```python
from build123d import *

# Parameters (mm, degrees)
BOSS_EXTRUDE1_DEPTH = 351.07
SKETCH2_W           = 4
SKETCH2_H           = 9
CUT_EXTRUDE1_DEPTH  = 1.5
BOSS_EXTRUDE2_DEPTH = 351.07


with BuildPart() as part:
    # Sketch1 → Boss-Extrude1 (new body)
    with BuildSketch(Plane(origin=(0, 0, 0), x_dir=(1, 0, 0), z_dir=(0, 1, 0))):
        with BuildLine():
            Line((-257.832794656, 48.5), (-160, 48.5))
            Line((-160, 48.5), (-160, 45.5))
            Line((-160, 45.5), (-257.832794656, 45.5))
            ThreePointArc((-257.832794656, 45.5), (-265.752584863, 42.515371489), (-269.732769794, 35.046153846))
            ThreePointArc((-269.732769794, 35.046153846), (-272, 0), (-269.732769794, -35.046153846))
            ThreePointArc((-269.732769794, -35.046153846), (-265.752584863, -42.515371489), (-257.832794656, -45.5))
            Line((-257.832794656, -45.5), (-160, -45.5))
            Line((-160, -45.5), (-160, -48.5))
            Line((-160, -48.5), (-257.832794656, -48.5))
            ThreePointArc((-257.832794656, -48.5), (-267.732532415, -44.769214361), (-272.707763578, -35.432692308))
            ThreePointArc((-272.707763578, -35.432692308), (-275, 0), (-272.707763578, 35.432692308))
            ThreePointArc((-272.707763578, 35.432692308), (-267.732532415, 44.769214361), (-257.832794656, 48.5))
        make_face()
    extrude(amount=BOSS_EXTRUDE1_DEPTH)

    # Sketch2 → Cut-Extrude1 (cut)
    with BuildSketch(Plane.XY.offset(-45.5)):
        with Locations((-252.832794656, 351.07)):
            Rectangle(SKETCH2_W, SKETCH2_H)
        with Locations((-185.832794656, 351.07)):
            Rectangle(SKETCH2_W, SKETCH2_H)
    cut_extrude1 = extrude(amount=-CUT_EXTRUDE1_DEPTH, mode=Mode.SUBTRACT)

    # Mirror1: Cut-Extrude1 across plane
    add(cut_extrude1.mirror(Plane.XY), mode=Mode.SUBTRACT)

    # Sketch3 → Boss-Extrude2 (add)
    with BuildSketch(Plane(origin=(0, 351.07, 0), x_dir=(1, 0, 0), z_dir=(0, 1, 0))):
        with BuildLine():
            Line((-176.5, -45.5), (-176.5, -32))
            ThreePointArc((-176.5, -32), (-175.914213562, -30.585786438), (-174.5, -30))
            Line((-174.5, -30), (-162, -30))
            ThreePointArc((-162, -30), (-161.292893219, -29.707106781), (-161, -29))
            Line((-161, -29), (-161, 29))
            ThreePointArc((-161, 29), (-161.292893219, 29.707106781), (-162, 30))
            Line((-162, 30), (-174.5, 30))
            ThreePointArc((-174.5, 30), (-175.914213562, 30.585786438), (-176.5, 32))
            Line((-176.5, 32), (-176.5, 45.5))
            Line((-176.5, 45.5), (-175.5, 45.5))
            Line((-175.5, 45.5), (-175.5, 32))
            ThreePointArc((-175.5, 32), (-175.207106781, 31.292893219), (-174.5, 31))
            Line((-174.5, 31), (-162, 31))
            ThreePointArc((-162, 31), (-160.585786438, 30.414213562), (-160, 29))
            Line((-160, 29), (-160, -29))
            ThreePointArc((-160, -29), (-160.585786438, -30.414213562), (-162, -31))
            Line((-162, -31), (-174.5, -31))
            ThreePointArc((-174.5, -31), (-175.207106781, -31.292893219), (-175.5, -32))
            Line((-175.5, -32), (-175.5, -45.5))
            Line((-175.5, -45.5), (-176.5, -45.5))
        make_face()
    extrude(amount=-BOSS_EXTRUDE2_DEPTH)


solid = part.part
```
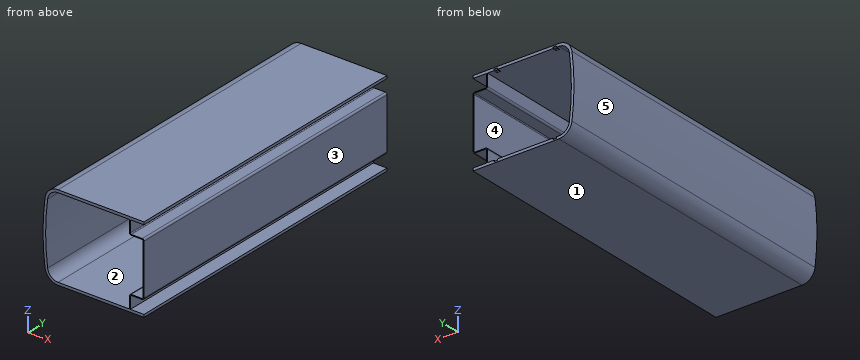
Design review of the part built by this model. Coordinates are the model's own, in mm. Face numbers are marked on the shaded views. A direction names the side the tool comes from. Coordinates: 2 decimals unless noted, no trailing zeros. Order: outer loops, then holes, each group sorted by start corner. A loop starts at its lowest first (then second) coordinate and runs counter-clockwise, first axis right, second up. Notation, with made-up numbers: (-10, 61) - (10, 61) arc R12 cw to (10, 70) - close; hole circle Ø7 at (87.25, 7.25). An arc over 180 degrees is marked (long way). Answer in a Markdown table with one row per item.
(1) Consider section B-B on z = 22.5. State the section outline as (x, y) points, plus the area to 3 significant figures.
Checked values:
| item | result |
|---|---|
| outline | (-274.08, 0) - (-271.07, 0) - (-271.07, 351.07) - (-274.08, 351.07) - close; (-161, 0) - (-160, 0) - (-160, 351.07) - (-161, 351.07) - close |
| area | 1,410 mm^2 |
(2) Consider section C-C on x = -213.5. State the section outline as (y, z) points.
Checked values:
| item | result |
|---|---|
| outline | (0, -48.5) - (351.07, -48.5) - (351.07, -45.5) - (0, -45.5) - close; (0, 45.5) - (351.07, 45.5) - (351.07, 48.5) - (0, 48.5) - close |
(3) For the marked faces 4 and 5, list the 3-axis set-ups (+Z, -Z, +X, -X, +Y, -Y) from which the entire face can be reached by the end or side of a thin tool; tool diameter is ignored.
Checked values:
| item | result |
|---|---|
| face 4 | +Y, -Y |
| face 5 | -X, +Y, -Y |
(4) Clearance check with flat-ended pins moving along their axes: pin 1 (2 mm diameter, centred on x = -261, y = 77, fed in from -Z); pin 2 (1.6 mm diameter, centred on y = 348.5, z = -46, fed in from -X); pin 3 (0.8 mm diameter, centred on y = 349, z = 46, fed in from -X). State where each tip first meets the part, or that it passes through.
Checked values:
| item | result |
|---|---|
| pin 1 | z = -48.34 |
| pin 2 | x = -267.22 |
| pin 3 | x = -266.7 |
(5) Wall thickness on line 1 along Z through (x, y) = (-245.5, 178); line 2 along X through (y, z) = (189.5, 35); line 3 along X through (y, z) = (211.5, 5.5) (3 decimals): over which ranges is each line inside the solid? List them lowest first. Write a range as from..to.
Checked values:
| item | result |
|---|---|
| line 1 | -48.5..-45.5, 45.5..48.5 |
| line 2 | -272.76..-269.74, -176.5..-175.5 |
| line 3 | -274.945..-271.944, -161..-160 |
(6) Consider section A-A on x = -168.5. State the section outline as (y, z) points, plus the area to 3 significant figures.
Checked values:
| item | result |
|---|---|
| outline | (0, -48.5) - (351.07, -48.5) - (351.07, -45.5) - (0, -45.5) - close; (0, -31) - (351.07, -31) - (351.07, -30) - (0, -30) - close; (0, 30) - (351.07, 30) - (351.07, 31) - (0, 31) - close; (0, 45.5) - (351.07, 45.5) - (351.07, 48.5) - (0, 48.5) - close |
| area | 2,810 mm^2 |
(7) The part is to be moulded in two halves that separate along Z. For the marked faces 1, 2 and 3, say which applies: released by +Z, released by -Z, zero draft, split by the parting line, or undercut.
Checked values:
| item | result |
|---|---|
| face 1 | released by -Z |
| face 2 | undercut |
| face 3 | zero draft |
